Drawing for the job (mm, zero at the part's lowest x, y, z). A direction names the side the tool comes from. Coordinates: 2 decimals unless noted, no trailing zeros. Write each loop counter-clockwise with the first axis right and the second up, starting at its lowest first coordinate (ties: lowest second). Pieces come first, ordered by that corner, then holes.
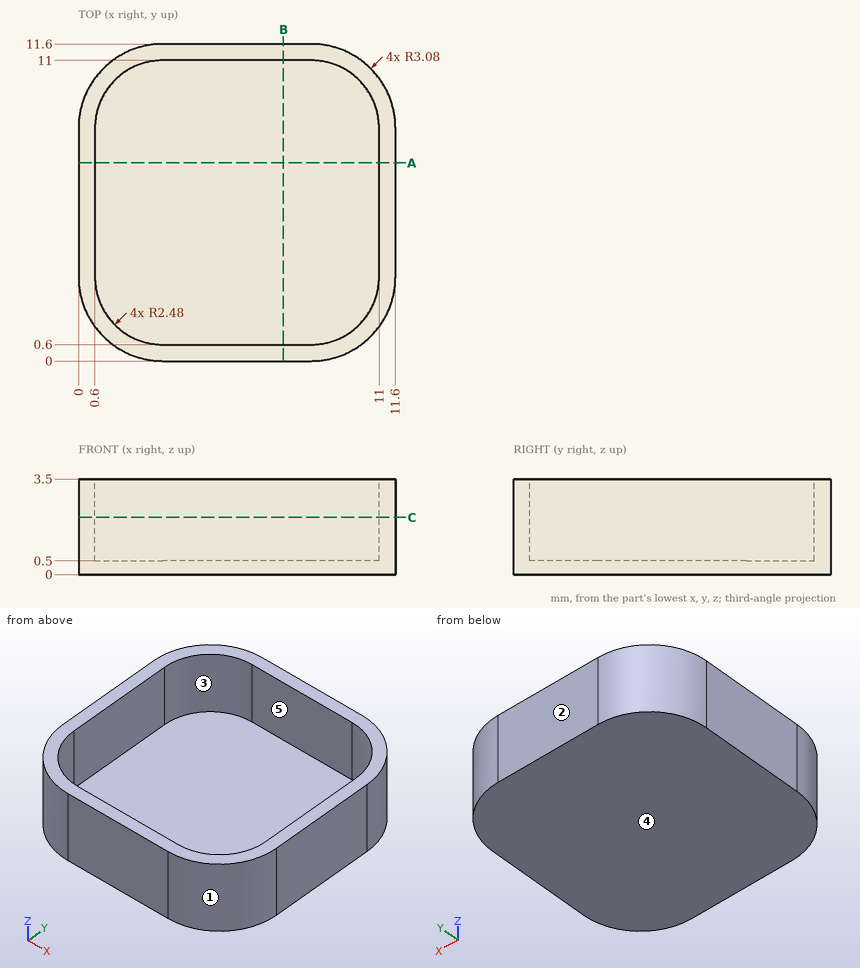
Item 1: Two-plate mould, pull along X, no slides. Class the marked faces 1, 2 and 3: +X half, -X half, draft (parallel to the pull), parting line (faces both ways), or undercut.
Item 2: Saw through at A-A, the plane y = 7.25. Write the cut outline in (x, z), and give its area (3 significant figures).
Item 3: Wall check: line 1 along Y through (x, z) = (4.25, 2.3); line 2 along Z through (x, y) = (2.75, 7). Give the ranges that are in metal, low to high.
Item 4: Saw through at C-C, the plane z = 2.1. Write the cut outline in (x, y), and give its area (3 significant figures).
Item 5: Which spindle directions (+Z, -Z, +X, -X, +Y, -Y) get a long thin tool onto all of the face, cutting with end or side? Do the marked faces 4 and 5. Say none if no direction does.
Item 6: Flat gauge pins, fed straight in: pin 1 Ø2 at (x, y) = (1.5, 4) entering from +Z; pin 2 Ø5 at (x, y) = (4.5, 4) entering from +Z; pin 3 Ø1.5 at (y, z) = (9.5, 2) entering from +X. Where does each tip first touch, or does it go through?
Working result:
1. face 1: +X half
1. face 2: draft
1. face 3: undercut
2. outline: (0, 0) - (11.6, 0) - (11.6, 3.5) - (11, 3.5) - (11, 0.5) - (0.6, 0.5) - (0.6, 3.5) - (0, 3.5) - close
2. area: 9.40 mm2
3. line 1: y = 0 to 0.6, 11 to 11.6
3. line 2: z = 0 to 0.5
4. outline: (0, 3.08) arc R3.08 ccw to (3.08, 0) - (8.52, 0) arc R3.08 ccw to (11.6, 3.08) - (11.6, 8.52) arc R3.08 ccw to (8.52, 11.6) - (3.08, 11.6) arc R3.08 ccw to (0, 8.52) - close; hole (0.6, 3.08) arc R2.48 ccw to (3.08, 0.6) - (8.52, 0.6) arc R2.48 ccw to (11, 3.08) - (11, 8.52) arc R2.48 ccw to (8.52, 11) - (3.08, 11) arc R2.48 ccw to (0.6, 8.52) - close
4. area: 23.5 mm2
5. face 4: -Z, +X, -X, +Y, -Y
5. face 5: +Z
6. pin 1: stops at z = 3.5
6. pin 2: stops at z = 0.5
6. pin 3: stops at x = 11.59
